For this review, take the finished solid that the model builds, in its own axes (mm). A direction names the side the tool comes from. Coordinates: 2 decimals unless noted, no trailing zeros. Loops run counter-clockwise (first coordinate to the right, second up) from the corner with the lowest first, then second, coordinate; pieces in that order, holes last. Notation, with made-up numbers: (3, 31) -> (14, 31) arc R17 ccw to (14, 56) -> close; hole circle Ø1 at (67, -14). An arc over 180 degrees is marked (long way). One line per item, written item: value.
from build123d import *

# Parameters (mm, degrees)
SKETCH1_R           = 10
BOSS_EXTRUDE1_DEPTH = 2
SKETCH2_W           = 8
SKETCH2_H           = 9.97
BOSS_EXTRUDE2_DEPTH = 2
SKETCH3_R           = 6
CUT_EXTRUDE1_DEPTH  = 3


with BuildPart() as part:
    # Sketch1 → Boss-Extrude1 (new body)
    with BuildSketch(Plane(origin=(0, 0, 0), x_dir=(1, 0, 0), z_dir=(0, 1, 0))):
        Circle(SKETCH1_R)
    extrude(amount=-BOSS_EXTRUDE1_DEPTH)

    # Sketch2 → Boss-Extrude2 (add)
    with BuildSketch(Plane(origin=(0, 0, 0), x_dir=(1, 0, 0), z_dir=(0, 1, 0))):
        with Locations((0, 14.15015139)):
            Rectangle(SKETCH2_W, SKETCH2_H)
    extrude(amount=-BOSS_EXTRUDE2_DEPTH)

    # Sketch3 → Cut-Extrude1 (cut, through all)
    with BuildSketch(Plane(origin=(0, 0, 0), x_dir=(1, 0, 0), z_dir=(0, 1, 0))):
        Circle(SKETCH3_R)
    extrude(amount=-CUT_EXTRUDE1_DEPTH, mode=Mode.SUBTRACT)


solid = part.part
1. For faces 5 (the flat face through (4, -1, -14)), 6 (the flat face through (0, -2, -8)), 7 (the flat face through (-4, -1, -14)), list the 3-axis set-ups (+Z, -Z, +X, -X, +Y, -Y) from which the entire face can be reached by the end or side of a thin tool; tool diameter is ignored.
Return value:
face 5: -Z, +X, +Y, -Y
face 6: +Z, -Z, +X, -X, -Y
face 7: -Z, -X, +Y, -Y
2. The part is to be moulded in two halves that separate along Z. For faces 1 (the cylindrical face through (-6, -1, 0)), 2 (the flat face through (0, 0, -8)), 3 (the cylindrical face through (0, -1, 10)), 4 (the flat face through (0, -1, -19.135)), say which applies: pulls with the +Z half, pulls with the -Z half, needs draft (parallel to the pull), parting line crosses it, or undercut.
Return value:
face 1: undercut
face 2: needs draft
face 3: parting line crosses it
face 4: pulls with the -Z half
3. Take a section at A-A, the plane z = 0. Give the boundary of the cut face in (x, y).
Return value:
outline: (-10, -2) -> (-6, -2) -> (-6, 0) -> (-10, 0) -> close; (6, -2) -> (10, -2) -> (10, 0) -> (6, 0) -> close
4. Insertion check: pin 1 Ø9.5 at (x, z) = (0, 0) entering from -Y; pin 2 Ø0.6 at (y, z) = (-0.5, -14.5) entering from +X. Each pin has a flat end and moves straight along its axis. Give the tip position at first contact, or say it passes through.
Return value:
pin 1: passes through
pin 2: stops at x = 4
5. To check wall thickness, follow probe 1 along Z at (x, y) = (0, -1.05); probe 2 along X at (y, z) = (-0.65, 0); probe 3 along X at (y, z) = (-1.7, 1.25). State the ranges of each line that lie inside material, in increasing order. Write a range as from..to.
Return value:
probe 1: z = -19.14..-6, 6..10
probe 2: x = -10..-6, 6..10
probe 3: x = -9.92..-5.87, 5.87..9.92
6. Take a section at D-D, the plane x = -6.75. Give the boundary of the cut face in (y, z), and give its area (3 significant figures).
Return value:
outline: (-2, -7.38) -> (0, -7.38) -> (0, 7.38) -> (-2, 7.38) -> close
area: 29.5 mm2
7. Take a section at B-B, the plane x = 0. Give the boundary of the cut face in (y, z), and give its area (3 significant figures).
Return value:
outline: (-2, -19.14) -> (0, -19.14) -> (0, -6) -> (-2, -6) -> close; (-2, 6) -> (0, 6) -> (0, 10) -> (-2, 10) -> close
area: 34.3 mm2
8. Take a section at C-C, the plane y = -1.7. Give the boundary of the cut face in (x, z), and give its area (3 significant figures).
Return value:
outline: (-4, -19.14) -> (4, -19.14) -> (4, -9.17) arc R10 ccw (long way) to (-4, -9.17) -> close; hole circle Ø12 at (0, 0)
area: 276 mm2
